Source: CAD feature listing. Evaluate the final solid. Frame: model axes, mm. Give positions to 0.01 mm unless a question says otherwise; leave off trailing zeros. Order: outer loops, then holes, each group sorted by start corner. A loop starts at its lowest first (then second) coordinate and runs counter-clockwise, first axis right, second up.
1) Section A-A, the plane x = 342.9. Return loops of the section in (y, z) (1 decimal).
2) First-contact query: P1, Ø3, axis at x = -311.15, z = 0, coming from the -Y side; P2, Ø3, axis at x = -441.325, z = 0, coming from the -Y side. Flat tips, straight axial feed; report the tip coordinate or a pass-through.
3) Material intervals for line 1 (Y direction, x = 209.5, z = -5.25) (3 decimals); line 2 (Z direction, x = 343, y = 11) (3 decimals); line 3 (X direction, y = 2.5, z = 10.25) (3 decimals), sorted ascending.
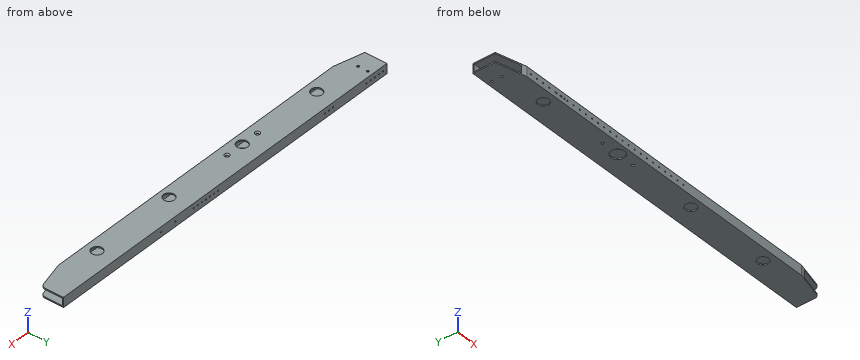
```python
from build123d import *

# Parameters (mm, degrees)
SKETCH1_W                                           = 1009.65
SKETCH1_H                                           = 76.2
SKETCH1_R                                           = 14.2875
BOSS_EXTRUDE2_DEPTH                                 = 12.7
SKETCH3_W                                           = 19.05
SKETCH3_H                                           = 69.85
CUT_EXTRUDE2_DEPTH                                  = 1011.448426442
CUT_EXTRUDE3_DEPTH                                  = 507.897475457
FILLET1_R                                           = 12.7
SKETCH9_R                                           = 1.7272
CUT_EXTRUDE5_DEPTH                                  = 6.35
SKETCH12_R                                          = 1.7272
CUT_EXTRUDE8_DEPTH                                  = 5.08
CSK_FOR_1_4_FLAT_HEAD_MACHINE_SCREW_100_D           = 6.7564
CSK_FOR_1_4_FLAT_HEAD_MACHINE_SCREW_100_CSINK_D     = 12.8778
CSK_FOR_1_4_FLAT_HEAD_MACHINE_SCREW_100_CSINK_ANGLE = 100
CUT_EXTRUDE9_START                                  = -6.35
SKETCH15_R                                          = 1.7272
CUT_EXTRUDE9_DEPTH                                  = 6.35
SKETCH16_R                                          = 17.4625
CUT_EXTRUDE10_DEPTH                                 = 3.81
F_1_4_0_25_DIAMETER_HOLE1_D                         = 6.35
F_10_32_TAPPED_HOLE2_D                              = 4.0386
F_10_32_TAPPED_HOLE2_DEPTH                          = 13.716
F_10_32_TAPPED_HOLE2_TIP                            = 1.213317848
F_10_32_TAPPED_HOLE3_D                              = 4.0386


with BuildPart() as part:
    # Sketch1 → Boss-Extrude2 (new, symmetric)
    with BuildSketch(Plane.XY):
        Rectangle(SKETCH1_W, SKETCH1_H)
        with Locations((114.3, -12.7)):
            Circle(SKETCH1_R, mode=Mode.SUBTRACT)
        with Locations((-342.9, -9.525)):
            Circle(SKETCH1_R, mode=Mode.SUBTRACT)
        with Locations((342.9, -9.525)):
            Circle(SKETCH1_R, mode=Mode.SUBTRACT)
        with Locations((-114.3, -12.7)):
            Circle(SKETCH1_R, mode=Mode.SUBTRACT)
    extrude(amount=BOSS_EXTRUDE2_DEPTH, both=True)

    # Sketch3 → Cut-Extrude2 (cut, through all)
    with BuildSketch(Plane(origin=(504.825, 0, 0), x_dir=(0, 0, -1), z_dir=(1, 0, 0))):
        Rectangle(SKETCH3_W, SKETCH3_H)
    extrude(amount=-CUT_EXTRUDE2_DEPTH, mode=Mode.SUBTRACT)

    # Sketch4 → Cut-Extrude3 (cut, through all)
    with BuildSketch(Plane.XY.offset(12.7)):
        Polygon((-504.825, -38.1), (-504.825, -19.05), (-428.625, -38.1), align=None)
        Polygon((428.625, -38.1), (504.825, -38.1), (504.825, -19.05), align=None)
    extrude(amount=-CUT_EXTRUDE3_DEPTH, mode=Mode.SUBTRACT)

    # Fillet1
    fillet1_edges = [part.edges().sort_by_distance(p)[0] for p in [
        (504.825, -19.05, 11.1125),
        (504.825, -19.05, -11.1125),
    ]]
    fillet(fillet1_edges, radius=FILLET1_R)

    # Sketch9 → Cut-Extrude5 (cut)
    with BuildSketch(Plane(origin=(0, 38.1, 0), x_dir=(1, 0, 0), z_dir=(0, 1, 0))):
        with Locations(Location((-492.125, 0, 0), (0, 0, 270))):
            Circle(SKETCH9_R)
        with Locations(Location((-441.325, 0, 0), (0, 0, 270))):
            Circle(SKETCH9_R)
        with Locations(Location((-479.425, 0, 0), (0, 0, 270))):
            Circle(SKETCH9_R)
        with Locations(Location((-466.725, 0, 0), (0, 0, 270))):
            Circle(SKETCH9_R)
        with Locations(Location((-454.025, 0, 0), (0, 0, 270))):
            Circle(SKETCH9_R)
    extrude(amount=-CUT_EXTRUDE5_DEPTH, mode=Mode.SUBTRACT)

    # Sketch12 → Cut-Extrude8 (cut)
    with BuildSketch(Plane(origin=(0, 38.1, 0), x_dir=(1, 0, 0), z_dir=(0, 1, 0))):
        with Locations(Location((98.425, 0, 0), (0, 0, 270))):
            Circle(SKETCH12_R)
        with Locations(Location((85.725, 0, 0), (0, 0, 270))):
            Circle(SKETCH12_R)
        with Locations(Location((73.025, 0, 0), (0, 0, 270))):
            Circle(SKETCH12_R)
        with Locations(Location((60.325, 0, 0), (0, 0, 270))):
            Circle(SKETCH12_R)
        with Locations(Location((47.625, 0, 0), (0, 0, 270))):
            Circle(SKETCH12_R)
        with Locations(Location((34.925, 0, 0), (0, 0, 270))):
            Circle(SKETCH12_R)
        with Locations(Location((22.225, 0, 0), (0, 0, 270))):
            Circle(SKETCH12_R)
    extrude(amount=-CUT_EXTRUDE8_DEPTH, mode=Mode.SUBTRACT)

    # CSK for 1/4 Flat Head Machine Screw (100)1 (through all)
    with Locations(Plane.XY.offset(12.7)):
        with Locations((-66.675, -12.7), (-161.925, -12.7)):
            CounterSinkHole(CSK_FOR_1_4_FLAT_HEAD_MACHINE_SCREW_100_D / 2, CSK_FOR_1_4_FLAT_HEAD_MACHINE_SCREW_100_CSINK_D / 2, counter_sink_angle=CSK_FOR_1_4_FLAT_HEAD_MACHINE_SCREW_100_CSINK_ANGLE)

    # Sketch15 → Cut-Extrude9 (cut)
    with BuildSketch(Plane(origin=(0, -38.1, 0), x_dir=(-1, 0, 0), z_dir=(0, -1, 0)).offset(CUT_EXTRUDE9_START)):
        with Locations(Location((415.925, 0, 0), (0, 0, 180))):
            Circle(SKETCH15_R)
        with Locations(Location((396.875, 0, 0), (0, 0, 180))):
            Circle(SKETCH15_R)
        with Locations(Location((377.825, 0, 0), (0, 0, 180))):
            Circle(SKETCH15_R)
        with Locations(Location((358.775, 0, 0), (0, 0, 180))):
            Circle(SKETCH15_R)
        with Locations(Location((339.725, 0, 0), (0, 0, 180))):
            Circle(SKETCH15_R)
        with Locations(Location((320.675, 0, 0), (0, 0, 180))):
            Circle(SKETCH15_R)
        with Locations(Location((301.625, 0, 0), (0, 0, 180))):
            Circle(SKETCH15_R)
        with Locations(Location((282.575, 0, 0), (0, 0, 180))):
            Circle(SKETCH15_R)
        with Locations(Location((263.525, 0, 0), (0, 0, 180))):
            Circle(SKETCH15_R)
        with Locations(Location((244.475, 0, 0), (0, 0, 180))):
            Circle(SKETCH15_R)
        with Locations(Location((225.425, 0, 0), (0, 0, 180))):
            Circle(SKETCH15_R)
        with Locations(Location((206.375, 0, 0), (0, 0, 180))):
            Circle(SKETCH15_R)
        with Locations(Location((187.325, 0, 0), (0, 0, 180))):
            Circle(SKETCH15_R)
        with Locations(Location((168.275, 0, 0), (0, 0, 180))):
            Circle(SKETCH15_R)
        with Locations(Location((149.225, 0, 0), (0, 0, 180))):
            Circle(SKETCH15_R)
        with Locations(Location((130.175, 0, 0), (0, 0, 180))):
            Circle(SKETCH15_R)
        with Locations(Location((111.125, 0, 0), (0, 0, 180))):
            Circle(SKETCH15_R)
        with Locations(Location((92.075, 0, 0), (0, 0, 180))):
            Circle(SKETCH15_R)
        with Locations(Location((73.025, 0, 0), (0, 0, 180))):
            Circle(SKETCH15_R)
        with Locations(Location((53.975, 0, 0), (0, 0, 180))):
            Circle(SKETCH15_R)
        with Locations(Location((34.925, 0, 0), (0, 0, 180))):
            Circle(SKETCH15_R)
        with Locations(Location((15.875, 0, 0), (0, 0, 180))):
            Circle(SKETCH15_R)
        with Locations(Location((-3.175, 0, 0), (0, 0, 180))):
            Circle(SKETCH15_R)
        with Locations(Location((-22.225, 0, 0), (0, 0, 270))):
            Circle(SKETCH15_R)
        with Locations(Location((-41.275, 0, 0), (0, 0, 180))):
            Circle(SKETCH15_R)
        with Locations(Location((-60.325, 0, 0), (0, 0, 270))):
            Circle(SKETCH15_R)
    extrude(amount=CUT_EXTRUDE9_DEPTH, mode=Mode.SUBTRACT)

    # Sketch16 → Cut-Extrude10 (cut)
    with BuildSketch(Plane(origin=(0, 0, -12.7), x_dir=(-1, 0, 0), z_dir=(0, 0, -1))):
        with Locations((114.3, -12.7)):
            Circle(SKETCH16_R)
    extrude(amount=-CUT_EXTRUDE10_DEPTH, mode=Mode.SUBTRACT)

    # 1/4 (0.25) Diameter Hole1 (through all)
    with Locations(Plane.XY.offset(12.7)):
        with Locations((-460.375, 25.4), (-460.375, 0)):
            Hole(F_1_4_0_25_DIAMETER_HOLE1_D / 2)

    # #10-32 Tapped Hole2
    with Locations(Plane(origin=(0, 38.1, 0), x_dir=(1, 0, 0), z_dir=(0, 1, 0))):
        with Locations((155.575, 0), (200.025, 0)):
            Hole(F_10_32_TAPPED_HOLE2_D / 2, depth=F_10_32_TAPPED_HOLE2_DEPTH)
            with Locations((0, 0, -(F_10_32_TAPPED_HOLE2_DEPTH + F_10_32_TAPPED_HOLE2_TIP / 2))):  # 118° drill point
                Cone(0, F_10_32_TAPPED_HOLE2_D / 2, F_10_32_TAPPED_HOLE2_TIP, mode=Mode.SUBTRACT)

    # #10-32 Tapped Hole3 (through all)
    with Locations(Plane(origin=(0, 38.1, 0), x_dir=(1, 0, 0), z_dir=(0, 1, 0))):
        with Locations((-336.55, 0), (-311.15, 0), (-323.85, 0)):
            Hole(F_10_32_TAPPED_HOLE3_D / 2)


solid = part.part
```
From the geometry:
1. outline: (-38.1, -12.7) - (-23.8, -12.7) - (-23.8, -9.5) - (-34.9, -9.5) - (-34.9, 9.5) - (-23.8, 9.5) - (-23.8, 12.7) - (-38.1, 12.7) - close; (4.8, -12.7) - (38.1, -12.7) - (38.1, 12.7) - (4.8, 12.7) - (4.8, 9.5) - (34.9, 9.5) - (34.9, -9.5) - (4.8, -9.5) - close
2. P1: passes through
2. P2: stops at y = -35.3
3. line 1: y = -38.1 to -34.925, 34.925 to 38.1
3. line 2: z = -12.7 to -9.525, 9.525 to 12.7
3. line 3: x = -504.825 to -462.332, -458.418 to -350.616, -335.184 to 335.184, 350.616 to 504.825
